Read the model definition and answer for the solid it produces. Units are mm, in the model's axes. A direction names the side the tool comes from. Coordinates: 2 decimals unless noted, no trailing zeros. Loops run counter-clockwise (first coordinate to the right, second up) from the corner with the lowest first, then second, coordinate; pieces in that order, holes last. Notation, with made-up numbers: (56.5, -38) -> (103.5, -38) arc R25 ccw to (103.5, -22) -> close; hole circle Ø10 at (27, 41). An arc over 180 degrees is marked (long way). Answer as a JSON object with one key per item and string values. Group by question number.
1) Consider probe 1 along Y at (x, z) = (37.5, 0.9); probe 2 along X at (y, z) = (67, 0.4); probe 3 along Y at (x, z) = (39.5, 2.85). Determine where each line is inside the solid, lowest interval first. Write a range as [from, to].
2) Flat-ended cylindrical pins translate along their axes: P1, Ø1.5, axis at y = 50, z = 1.5, coming from the -X side; P2, Ø1, axis at x = 13, z = 2, coming from the -Y side; P3, Ø1, axis at x = 15.5, z = 1, coming from the -Y side. Find the tip coordinate at first contact, or state that the pin passes through.
3) Section D-D, the plane y = 16 is taken. Give the vertices of the cut face in (x, z).
4) Section A-A, the plane x = 37.5 is taken. Give the vertices of the cut face in (y, z).
5) Section B-B, the plane y = 62 is taken. Give the vertices of the cut face in (x, z), plus the area to 3 significant figures.
6) Which of the six approach directions +Z, -Z, +X, -X, +Y, -Y give full straight-line access (tool end or side, diameter ignored) to faces 1 (the face through (34.496, 73.072, 1.479)), 2 (the face through (37, 30, 0))?
7) Section C-C, the plane z = 2 is taken. Give the vertices of the cut face in (x, y), plus the area to 3 significant figures.
8) Determine the mould class of faces 3 (the face through (35.29, 39.53, 1.48)), 4 (the face through (37, 30, 3)) for opening direction Y: released by +Y, released by -Y, zero draft, split by the parting line, or undercut.
from build123d import *

# Parameters (mm, degrees)
F0_R     = 3
F1_DEPTH = 3


with BuildPart() as f1:
    # F0 (on Top) → F1 (new body)
    with BuildSketch(Plane.XY):
        with BuildLine():
            ThreePointArc((32.235098, 74.628571), (12.915287, 9.183187), (75, 37.5))
            ThreePointArc((75, 37.5), (65.816813, 62.084713), (42.764902, 74.628571))
            ThreePointArc((42.764902, 74.628571), (40.513824, 73.11211), (41.789806, 70.716514))
            ThreePointArc((41.789806, 70.716514), (47.808281, 66.108235), (50.090155, 58.879726))
            ThreePointArc((50.090155, 58.879726), (30.271491, 48.571444), (33.210194, 70.716514))
            ThreePointArc((33.210194, 70.716514), (34.486176, 73.11211), (32.235098, 74.628571))
        make_face()
        with Locations((37.5, 37.5)):
            Circle(F0_R, mode=Mode.SUBTRACT)
    extrude(amount=F1_DEPTH)


solid = f1.part
Determined:
{
 "1": {"probe 1": "[0, 34.5], [40.5, 46.29]", "probe 2": "[14.35, 27.88], [47.12, 60.65]", "probe 3": "[0.05, 35.26], [39.74, 46.45]"},
 "2": {"P1": "x = 1.89", "P2": "y = 8.69", "P3": "y = 6.78"},
 "3": {"outline": "(6.78, 0) -> (68.22, 0) -> (68.22, 3) -> (6.78, 3) -> close"},
 "4": {"outline": "(0, 0) -> (34.5, 0) -> (34.5, 3) -> (0, 3) -> close; (40.5, 0) -> (46.29, 0) -> (46.29, 3) -> (40.5, 3) -> close"},
 "5": {"outline": "(9.11, 0) -> (25.3, 0) -> (25.3, 3) -> (9.11, 3) -> close; (49.7, 0) -> (65.89, 0) -> (65.89, 3) -> (49.7, 3) -> close", "area": "97.2 mm²"},
 "6": {"face 1": "+Z, -Z", "face 2": "-Z, +X, -X, +Y, -Y"},
 "7": {"outline": "(32.24, 74.63) arc R37.5 ccw (long way) to (75, 37.5) arc R37.5 ccw to (42.76, 74.63) arc R2.03 ccw to (41.79, 70.72) arc R12.59 cw to (50.09, 58.88) arc R12.59 cw (long way) to (33.21, 70.72) arc R2.03 ccw to start; hole circle Ø6 at (37.5, 37.5)", "area": "3,870 mm²"},
 "8": {"face 3": "undercut", "face 4": "zero draft"}
}
